from build123d import *

# Parameters (mm, degrees)
BOSS_EXTRUDE1_DEPTH      = 2.5
BOSS_EXTRUDE1_DEPTH_BACK = 1.5
SKETCH2_R                = 1.5875
CUT_EXTRUDE1_DEPTH       = 44.756449915
CUT_EXTRUDE3_DEPTH       = 59.296841331
SKETCH4_W                = 4.2
SKETCH4_H                = 22.2
BOSS_EXTRUDE2_DEPTH      = 32.1
SKETCH6_W                = 23.3
SKETCH6_H                = 12.95
CUT_EXTRUDE4_DEPTH       = 4.2
SKETCH7_W                = 4.2
SKETCH7_H                = 22.2
BOSS_EXTRUDE3_DEPTH      = 5
CUT_EXTRUDE5_DEPTH       = 3.7
FILLET1_R                = 5
F_2_0MM_DOWEL_HOLE1_D    = 2.2
SKETCH12_W               = 37.1
SKETCH12_H               = 2.25
CUT_EXTRUDE6_DEPTH       = 4.2
FILLET3_R                = 2
CUT_EXTRUDE7_REACH       = 51.552


with BuildPart() as part:
    # Sketch1 → Boss-Extrude1 (new, two sides: drawn at the far end of the back side and taken through both)
    with BuildSketch(Plane.XY.offset(-BOSS_EXTRUDE1_DEPTH_BACK)):
        with BuildLine():
            Line((-33.54, 5), (33.54, 5))
            ThreePointArc((33.54, 5), (38.423518139, 1.072963462), (35.635934611, -4.539499764))
            Line((35.635934611, -4.539499764), (2.434033336, -19.869165506))
            ThreePointArc((2.434033336, -19.869165506), (0.357155817, -20.329629424), (-1.723171376, -19.885010467))
            Line((-1.723171376, -19.885010467), (-35.601270101, -4.555344726))
            ThreePointArc((-35.601270101, -4.555344726), (-38.42757218, 1.054342537), (-33.54, 5))
        make_face()
    extrude(amount=BOSS_EXTRUDE1_DEPTH + BOSS_EXTRUDE1_DEPTH_BACK)

    # Sketch2 → Cut-Extrude1 (cut, through all)
    with BuildSketch(Plane.XY.offset(2.5)):
        with Locations((-33.54, 0)):
            Circle(SKETCH2_R)
        with Locations((33.54, 0)):
            Circle(SKETCH2_R)
        with Locations((0.338098725, -15.329665742)):
            Circle(SKETCH2_R)
    extrude(amount=-CUT_EXTRUDE1_DEPTH, mode=Mode.SUBTRACT)

    # Sketch3 → Cut-Extrude3 (cut, through all)
    with BuildSketch(Plane.ZY.offset(16.04)):
        Polygon((-1.5, -4.555344726), (-1.5, -19.885010467), (2.5, -19.885010467), (2.5, -4.555344726), (2.5, 5), (-1.5, 5), align=None)
    extrude(amount=CUT_EXTRUDE3_DEPTH, mode=Mode.SUBTRACT)

    # Sketch4 → Boss-Extrude2 (add)
    with BuildSketch(Plane.ZY.offset(12.34)):
        with Locations((4.6, 0)):
            Rectangle(SKETCH4_W, SKETCH4_H)
    extrude(amount=BOSS_EXTRUDE2_DEPTH)

    # Sketch6 → Cut-Extrude4 (cut)
    with BuildSketch(Plane(origin=(0, 0, 2.5), x_dir=(-1, 0, 0), z_dir=(0, 0, -1))):
        with Locations((28.29, -0.125)):
            Rectangle(SKETCH6_W, SKETCH6_H)
    extrude(amount=-CUT_EXTRUDE4_DEPTH, mode=Mode.SUBTRACT)

    # Sketch7 → Boss-Extrude3 (add)
    with BuildSketch(Plane(origin=(-12.34, 0, 0), x_dir=(0, 0, -1), z_dir=(1, 0, 0))):
        with Locations((-4.6, 0)):
            Rectangle(SKETCH7_W, SKETCH7_H)
    extrude(amount=BOSS_EXTRUDE3_DEPTH)

    # Sketch8 → Cut-Extrude5 (cut)
    with BuildSketch(Plane.ZY.offset(12.34)):
        Polygon((2.5, -13.406719018), (2.5, -11.1), (2.5, 5), (-1.5, 5), (-1.5, -13.406719018), (-1.5, -19.885010467), (2.5, -19.885010467), align=None)
    extrude(amount=CUT_EXTRUDE5_DEPTH, mode=Mode.SUBTRACT)

    # Fillet1
    fillet1_edges = [part.edges().sort_by_distance(p)[0] for p in [
        (-44.44, -11.1, 4.6),
    ]]
    fillet(fillet1_edges, radius=FILLET1_R)

    # Fillet2
    # a fillet whose section is not a circle: 13, 9 mm, written as the material it takes off along each edge
    with BuildSketch(Plane(origin=(-12.34, -15.080950022, 2.5), x_dir=(0, 1, 0), z_dir=(0, 0, -1))) as fillet2_piece_1:
        with BuildLine():
            Bezier((3.996072697, 0), (0, 0), (-4.203547809, 9.289713818), weights=[1, 0.840313638, 1])
            Line((-4.203547809, 9.289713818), (0, 0))
            Line((0, 0), (3.996072697, 0))
        make_face()
    extrude(amount=29.491248131, mode=Mode.SUBTRACT)

    # Ø2.0mm Dowel Hole1 (through all)
    with Locations(Plane.XY.offset(6.7)):
        with Locations((-42.3, -0.06), (-14.49, -0.06)):
            Hole(F_2_0MM_DOWEL_HOLE1_D / 2)

    # Sketch12 → Cut-Extrude6 (cut)
    with BuildSketch(Plane.XY.offset(6.7)):
        with Locations((-25.89, 9.975)):
            Rectangle(SKETCH12_W, SKETCH12_H)
    extrude(amount=-CUT_EXTRUDE6_DEPTH, mode=Mode.SUBTRACT)

    # Fillet3
    fillet3_edges = [part.edges().sort_by_distance(p)[0] for p in [
        (-44.44, 8.85, 4.6),
    ]]
    fillet(fillet3_edges, radius=FILLET3_R)

    # Sketch13 → Cut-Extrude7 (cut, up to next)
    with BuildSketch(Plane.XY.offset(6.7), mode=Mode.PRIVATE) as cut_extrude7_sk1:
        Polygon((-7.34, 8.85), (-7.34, 7.85), (-24.64, 8.85), align=None)
    cut_extrude7_tool1 = extrude(cut_extrude7_sk1.sketch, amount=-CUT_EXTRUDE7_REACH, mode=Mode.PRIVATE) & part.part
    add(cut_extrude7_tool1.solids().sort_by_distance((-13.106667, 8.516667, 6.7))[0], mode=Mode.SUBTRACT)


solid = part.part
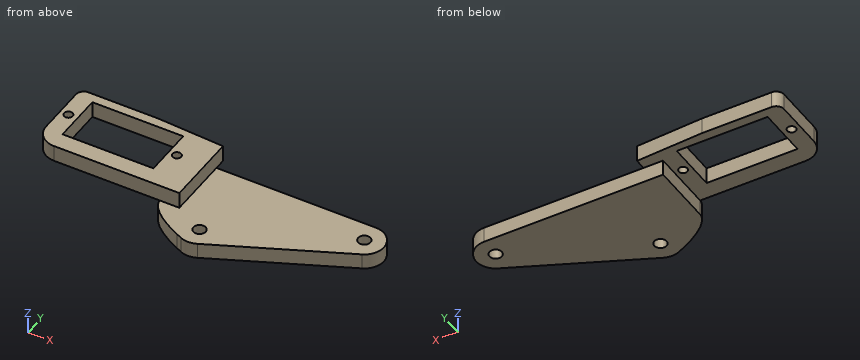
Part model, mm, in its own coordinate system. Coordinates: 2 decimals unless noted, no trailing zeros. Loops run counter-clockwise (first coordinate to the right, second up) from the corner with the lowest first, then second, coordinate; pieces in that order, holes last. Notation, with made-up numbers: M -38,76.25 L 13,76.25 A12 ccw 13,98.25 Z; hole C 76,3.25 d2. An arc over 180 degrees is marked long. Use a Markdown table: item, result. Add a question column.
Q1. Probe L1, parallel to X at y = 6, z = 6.25; L2, parallel to Z at x = 2.5, y = 4; L3, parallel to Z at x = -33, y = -9.25. List the from-to ranges inside material, lowest first.
Q2. Cut at C-C (x = 22.5). Write the cut outline in (y, z).
Q3. Cut at A-A (x = -14.49). Write the cut outline in (y, z).
Q4. Pin check, flat tips, straight feed: P1, Ø3, axis at x = 18.5, z = 0.5, coming from the +Y side; P2, Ø5, axis at x = 0.34, y = -15.33, coming from the +Z side; P3, Ø3.5, axis at x = -22.5, z = 5.5, coming from the -Y side; P4, Ø3.5, axis at x = -42.3, y = -0.06, coming from the +Z side. Stop position of each tip, or through.
Q5. Cut at D-D (z = 1). Give the number of separate pieces and of enclosed holes in the cut face, and give its area (3 significant figures).
Q6. Cut at B-B (y = 3.25). Write the cut outline in (x, z), and give its area (3 significant figures).
Worked out:
| question | item | result |
|---|---|---|
| 1 | L1 | x = -44.44 to -39.94, -16.64 to -7.34 |
| 1 | L2 | z = -1.5 to 2.5 |
| 1 | L3 | z = 2.5 to 6.7 |
| 2 | outline | M -10.6,-1.5 L 5,-1.5 L 5,2.5 L -10.6,2.5 Z |
| 3 | outline | M -11.1,2.5 L -1.16,2.5 L -1.16,6.7 L -11.1,6.7 Z; M 1.04,2.5 L 8.26,2.5 L 8.26,6.7 L 1.04,6.7 Z |
| 4 | P1 | stops at y = 5 |
| 4 | P2 | stops at z = 2.5 |
| 4 | P3 | stops at y = -11.1 |
| 4 | P4 | stops at z = 6.7 |
| 5 | separate pieces | 1 |
| 5 | enclosed holes | 2 |
| 5 | area | 910 mm2 |
| 6 | outline | M -44.44,2.5 L -39.94,2.5 L -39.94,6.7 L -44.44,6.7 Z; M -16.64,2.5 L -12.34,2.5 L -12.34,-1.5 L 37.34,-1.5 L 37.34,2.5 L -7.34,2.5 L -7.34,6.7 L -16.64,6.7 Z |
| 6 | area | 257 mm2 |
